Autodesk Inventor part; units mm, degrees
ref_plane "YZ Plane" through (0, 0, 0) normal (1, 0, 0) x (0, 1, 0)
ref_plane "XZ Plane" through (0, 0, 0) normal (0, 1, 0) x (-1, 0, 0)
ref_plane "XY Plane" through (0, 0, 0) normal (0, 0, 1) x (1, 0, 0)
sketch "Sketch4" plane through (0, 0, 0) normal (0, 1, 0) x (-1, 0, 0)
  circle A0 centre (0, 0) radius 38.735
  circle A1 centre (0, 0) radius 50.8
  dimension "d9" = 77.47
  dimension "d10" = 101.6
extrude "Extrusion2" add sketch "Sketch4" along normal blind 6.35
sketch "Sketch5" plane through (0, 6.35, 0) normal (0, 1, 0) x (1, 0, 0)
  circle A0 centre (0, -44.45) radius 2.667
  circle A1 centre (38.4948, -22.225) radius 2.667
  circle A2 centre (38.4948, 22.225) radius 2.667
  circle A3 centre (0, 44.45) radius 2.667
  circle A4 centre (-38.4948, 22.225) radius 2.667
  circle A5 centre (-38.4948, -22.225) radius 2.667
  point P0 (0, 0)
  dimension "d13" = 5.334
  dimension "d16" = 360
extrude "Extrusion3" cut sketch "Sketch5" against normal blind 6.35
sketch "Sketch7" plane through (0, 6.35, 0) normal (0, 1, 0) x (1, 0, 0)
  line L0 (50.8, 12.7) -> (81.788, 12.7)
  line L1 (81.788, 12.7) -> (81.788, -12.7)
  line L2 (81.788, -12.7) -> (50.8, -12.7)
  line L3 (50.8, -12.7) -> (50.8, 12.7)
  line L4 (-50.8, 12.7) -> (-81.788, 12.7)
  line L5 (-81.788, 12.7) -> (-81.788, -12.7)
  line L6 (-81.788, -12.7) -> (-50.8, -12.7)
  line L7 (-50.8, -12.7) -> (-50.8, 12.7)
  point P0 (0, 0)
  dimension "d50" = 30.988
  dimension "d51" = 25.4
  dimension "d52" = 30.988
extrude "Extrusion4" add sketch "Sketch7" against normal blind 6.35
sketch "Sketch8" plane through (0, 6.35, 0) normal (0, 1, 0) x (1, 0, 0)
  line L0 (-123.5202, 12.7) -> (-50.8, 12.7)
  line L1 (-60.9386, 12.7) -> (-45.3133, 12.7)
  line L2 (-45.3133, 12.7) -> (-45.3133, -12.7)
  line L3 (-45.3133, -12.7) -> (-60.9386, -12.7)
  line L4 (-60.9386, -12.7) -> (-60.9386, 12.7)
  line L5 (57.1886, 12.7) -> (43.7508, 12.7)
  line L6 (43.7508, 12.7) -> (43.7508, -12.7)
  line L7 (43.7508, -12.7) -> (57.1886, -12.7)
  line L8 (57.1886, -12.7) -> (57.1886, 12.7)
  point P0 (0, 0)
extrude "Extrusion5" add sketch "Sketch8" against normal blind 6.35
sketch "Sketch9" plane through (0, 6.35, 0) normal (0, 1, 0) x (1, 0, 0)
  line L0 (111.76, 12.7) -> (111.76, -12.7)
  line L1 (81.788, 12.7) -> (81.788, -12.7)
  circle A0 centre (81.788, 0) radius 12.7
  line L2 (-81.788, 12.7) -> (-81.788, -12.7)
  circle A1 centre (-81.788, 0) radius 12.7
  point P0 (0, 0)
  point P1 (-111.7602, 0)
  point P2 (-111.76, -12.7)
extrude "Extrusion6" add sketch "Sketch9" against normal blind 6.35
sketch "Sketch10" plane through (0, 6.35, 0) normal (0, 1, 0) x (1, 0, 0)
  circle A0 centre (81.28, 0) radius 3.175
  circle A1 centre (91.3638, 0) radius 1.27
  circle A2 centre (76.2381, 8.7328) radius 1.27
  circle A3 centre (76.2381, -8.7328) radius 1.27
  circle A4 centre (-81.28, 0) radius 3.175
  circle A5 centre (-91.3638, 0) radius 1.27
  circle A6 centre (-76.2381, -8.7328) radius 1.27
  circle A7 centre (-76.2381, 8.7328) radius 1.27
  point P0 (0, 0)
  dimension "d53" = 6.35
  dimension "d54" = 2.54
  dimension "d57" = 360
  dimension "d59" = 6.35
  dimension "d60" = 2.54
  dimension "d63" = 360
extrude "Extrusion7" cut sketch "Sketch10" against normal blind 6.35
sketch "Sketch11" plane through (0, 6.35, 0) normal (0, 1, 0) x (1, 0, 0)
  arc A0 (-81.788, 12.7) -> (-81.788, -12.7) centre (-81.788, 0) ccw
  line L0 (-94.488, 0) -> (-81.788, 0)
  line L1 (-81.788, 0) -> (-81.788, -12.7)
  line L2 (-81.788, -12.7) -> (-94.488, -12.7)
  line L3 (-94.488, -12.7) -> (-94.488, 0)
  arc A1 (81.788, -12.7) -> (81.788, 12.7) centre (81.788, 0) ccw
  line L4 (94.488, 0) -> (81.788, 0)
  line L5 (81.788, 0) -> (81.788, -12.7)
  line L6 (81.788, -12.7) -> (94.488, -12.7)
  line L7 (94.488, -12.7) -> (94.488, 0)
  point P0 (0, 0)
extrude "Extrusion8" add sketch "Sketch11" against normal blind 6.35 contours A0 L2 L3 | A1 L7 L6
sketch "Sketch12" plane through (0, 6.35, 0) normal (0, 1, 0) x (1, 0, 0)
  line L0 (-49.1869, -12.7) -> (-94.488, -12.7)
  line L1 (-81.28, -12.7) -> (-60.96, -12.7)
  line L2 (-60.96, -12.7) -> (-60.96, -19.05)
  line L3 (-60.96, -19.05) -> (-81.28, -19.05)
  line L4 (-81.28, -19.05) -> (-81.28, -12.7)
  line L5 (94.488, -12.7) -> (49.1869, -12.7)
  line L6 (81.28, -12.7) -> (60.96, -12.7)
  line L7 (60.96, -12.7) -> (60.96, -19.05)
  line L8 (60.96, -19.05) -> (81.28, -19.05)
  line L9 (81.28, -19.05) -> (81.28, -12.7)
  point P0 (0, 0)
  dimension "d67" = 20.32
  dimension "d68" = 6.35
  dimension "d69" = 20.32
extrude "Extrusion9" add sketch "Sketch12" against normal blind 6.35
properties part number "middle plate2"
Can you work these out from the model? Positions are in its coordinate system, mm. A direction names the side the tool comes from. Give positions to 0.01 mm unless a question says otherwise; leave off trailing zeros. Order: outer loops, then holes, each group sorted by start corner. A loop starts at its lowest first (then second) coordinate and runs counter-clockwise, first axis right, second up. Notation, with made-up numbers: M 76,84 L 111,84 A18 ccw 111,114 Z; hole C -16,-16.5 d8. An arc over 180 degrees is marked long. Write item = value, one per line. Start each with the question number.
Q1. Suppose I cut it at A-A (x = 0). Write out the boundary of the cut face in (y, z) (3 decimals).
Q2. Will these pins go through, and if not, where does the flat tip stop? pin 1 Ø3 at (x, z) = (76.24, -8.73) entering from -Y; pin 2 Ø3 at (x, y) = (-43, 2) entering from +Z; pin 3 Ø3 at (y, z) = (3, 15) entering from +X; pin 4 Ø1.9 at (x, y) = (-75.5, 2.5) entering from +Z.
Q3. We'd pull the mould along Z, two halves only. Please class faces 6 (the cylindrical face through (-40.61, 3.22, 23.85)), 7 (the flat face through (-88, 3, 12.7)), 8 (the cylindrical face through (90.87, 3.22, -8.88)): pulls with the +Z half, pulls with the -Z half, needs draft (parallel to the pull), parting line crosses it, or undercut.
Q4. I need wall thicknesses on probe 1 along X at (y, z) = (2.25, 20); probe 2 along X at (y, z) = (5.5, 27); probe 3 along X at (y, z) = (5.5, -26). Which ranges of each line are inside material? Lowest first, please. Write a range as [from, to].
Q5. Suppose I cut it at D-D (z = -28). Write out the boundary of the cut face in (x, y), plus the area to 3 significant figures.
Q6. Suppose I cut it at C-C (y = 2). Count the separate pieces of the cut face and the enclosed holes in it, plus the area to 3 significant figures.
Q7. For faces 1 (the flat face through (-81.28, 3, 16)), 2 (the flat face through (-60.96, 3, 16)), 3 (the cylindrical face through (36.38, 3.22, 23.85)), 4 (the flat face through (88, 3, 12.7)), 5 (the flat face through (66, 3, -12.7)), which set-ups out of +Z, -Z, +X, -X, +Y, -Y let a thin tool reach every point of the face, with its end or its side?
Q8. Suppose I cut it at B-B (z = 29). Write out the boundary of the cut face in (x, y).
Check result:
q1.outline = M 0,-50.8 L 6.35,-50.8 L 6.35,-47.117 L 0,-47.117 Z; M 0,-41.783 L 6.35,-41.783 L 6.35,-38.735 L 0,-38.735 Z; M 0,38.735 L 6.35,38.735 L 6.35,41.783 L 0,41.783 Z; M 0,47.117 L 6.35,47.117 L 6.35,50.8 L 0,50.8 Z
q2.pin_1 = 0
q2.pin_2 = 29.3
q2.pin_3 = 81.28
q2.pin_4 = 19.05
q3.face_6 = undercut
q3.face_7 = pulls with the +Z half
q3.face_8 = pulls with the -Z half
q4.probe_1 = [-46.7, -39.97], [-37.02, -33.17], [33.17, 37.02], [39.97, 46.7]
q4.probe_2 = [-43.03, -27.77], [27.77, 43.03]
q4.probe_3 = [-43.64, -28.71], [28.71, 43.64]
q5.outline = M -42.39,0 L -26.77,0 L -26.77,6.35 L -42.39,6.35 Z; M 26.77,0 L 42.39,0 L 42.39,6.35 L 26.77,6.35 Z
q5.area = 198 mm2
q6.separate_pieces = 1
q6.enclosed_holes = 15
q6.area = 5,600 mm2
q7.face_1 = +Z, -X, +Y, -Y
q7.face_2 = +Z, +Y, -Y
q7.face_3 = +Y, -Y
q7.face_4 = +Z, +X, +Y, -Y
q7.face_5 = -Z, +X, +Y, -Y
q8.outline = M -41.71,0 L -25.68,0 L -25.68,6.35 L -41.71,6.35 Z; M 25.68,0 L 41.71,0 L 41.71,6.35 L 25.68,6.35 Z
